Can you work these out from the model? Positions are in its coordinate system, mm. A direction names the side the tool comes from. Give positions to 0.01 mm unless a question says otherwise; leave off trailing zeros. Loops run counter-clockwise (first coordinate to the right, second up) from the corner with the lowest first, then second, coordinate; pieces in that order, holes last. Notation, with made-up numbers: (44, 63) - (51, 63) arc R16 cw to (51, 76) - close; hole circle Ø7 at (31, 9). An arc over 180 degrees is marked (long way). Answer in a Markdown table with one row per item.
from build123d import *

# Parameters (mm, degrees)
BOSS_EXTRUDE1_DEPTH  = 21
SKETCH2_R            = 1.825
CUT_EXTRUDE1_DEPTH   = 4
SKETCH3_W            = 7.5
SKETCH3_H            = 11.75
CUT_EXTRUDE2_DEPTH   = 13
FILLET1_R            = 4
SKETCH5_R            = 1.825
CUT_EXTRUDE3_DEPTH   = 41.522370365
FILLET1_OF_MIRROR1_R = 4


with BuildPart() as part:
    # Sketch1 → Boss-Extrude1 (new body)
    with BuildSketch(Plane(origin=(0, 0, 0), x_dir=(1, 0, 0), z_dir=(0, 1, 0))):
        Polygon((-24.5, 0), (-24.5, 12.75), (0, 12.75), (0, 15.75), (-35, 15.75), (-35, 0), align=None)
    boss_extrude1 = extrude(amount=BOSS_EXTRUDE1_DEPTH)

    # Sketch2 → Cut-Extrude1 (cut)
    with BuildSketch(Plane.XY):
        with Locations((-31.25, 7)):
            Circle(SKETCH2_R)
    cut_extrude1 = extrude(amount=-CUT_EXTRUDE1_DEPTH, mode=Mode.SUBTRACT)

    # Sketch3 → Cut-Extrude2 (cut)
    with BuildSketch(Plane.XZ):
        with Locations((-31.25, -9.875)):
            Rectangle(SKETCH3_W, SKETCH3_H)
    cut_extrude2 = extrude(amount=-CUT_EXTRUDE2_DEPTH, mode=Mode.SUBTRACT)

    # Fillet1
    fillet1_edges = [part.edges().sort_by_distance(p)[0] for p in [
        (-35, 17, -15.75),
    ]]
    fillet(fillet1_edges, radius=FILLET1_R)

    # Sketch5 → Cut-Extrude3 (cut, through all)
    with BuildSketch(Plane.XZ.offset(-13)):
        with Locations(Location((-31, -11.75, 0), (0, 0, 270))):
            Circle(SKETCH5_R)
    cut_extrude3 = extrude(amount=-CUT_EXTRUDE3_DEPTH, mode=Mode.SUBTRACT)

    # Mirror1: Boss-Extrude1, Cut-Extrude1, Cut-Extrude2, Cut-Extrude3 across plane
    add(boss_extrude1.mirror(Plane(origin=(0, 21, 0), x_dir=(0, 0, 1), z_dir=(-1, 0, 0))))
    add(cut_extrude1.mirror(Plane(origin=(0, 21, 0), x_dir=(0, 0, 1), z_dir=(-1, 0, 0))), mode=Mode.SUBTRACT)
    add(cut_extrude2.mirror(Plane(origin=(0, 21, 0), x_dir=(0, 0, 1), z_dir=(-1, 0, 0))), mode=Mode.SUBTRACT)
    add(cut_extrude3.mirror(Plane(origin=(0, 21, 0), x_dir=(0, 0, 1), z_dir=(-1, 0, 0))), mode=Mode.SUBTRACT)

    # Fillet1 of Mirror1
    fillet1_of_mirror1_edges = [part.edges().sort_by_distance(p)[0] for p in [
        (35, 17, -15.75),
    ]]
    fillet(fillet1_of_mirror1_edges, radius=FILLET1_OF_MIRROR1_R)


solid = part.part
Q1. If we mould it in two halves opening along X, with no side actions, what happens to faces 1 (the face through (30, 10, 0)), 2 (the face through (29.77, 16.94, -10.4)), 3 (the face through (35, 13, -3))? For each: released by +X, released by -X, zero draft, split by the parting line, or undercut.
Checked values:
| item | result |
|---|---|
| face 1 | zero draft |
| face 2 | undercut |
| face 3 | released by +X |
Q2. Imagine slicing it at A-A, the plane z = -2.5. Write out the boundary of the cut face in (x, y) (3 decimals), and give its area (3 significant figures).
Checked values:
| item | result |
|---|---|
| outline | (-35, 0) - (-24.5, 0) - (-24.5, 21) - (-35, 21) - close; (24.5, 0) - (35, 0) - (35, 21) - (24.5, 21) - close; hole circle Ø3.65 at (-31.25, 7); hole circle Ø3.65 at (31.25, 7) |
| area | 420 mm² |
Q3. For pin 1 (2 mm diameter, centred on x = 32, z = -9.5, fed in from -Y); pin 2 (4.5 mm diameter, centred on x = 31.25, y = 7, fed in from -Z); pin 3 (8 mm diameter, centred on x = 7, y = 5.5, fed in from +Z); pin 4 (1 mm diameter, centred on x = 14.5, z = -12, fed in from +Y), each with a flat end and sliding along its axis, tell me the tip position at first contact or that it passes through.
Checked values:
| item | result |
|---|---|
| pin 1 | stops at y = 13 |
| pin 2 | stops at z = -4 |
| pin 3 | stops at z = -12.75 |
| pin 4 | passes through |
Q4. Imagine slicing it at C-C, the plane y = 10.25. Write out the boundary of the cut face in (x, z), and give its area (4 significant figures).
Checked values:
| item | result |
|---|---|
| outline | (-35, -4) - (-27.5, -4) - (-27.5, -15.75) - (27.5, -15.75) - (27.5, -4) - (35, -4) - (35, 0) - (24.5, 0) - (24.5, -12.75) - (-24.5, -12.75) - (-24.5, 0) - (-35, 0) - close |
| area | 301.5 mm² |
Q5. If I drill on line 1 (X direction, y = 16.5, z = -11.75) (3 decimals); line 2 (Y direction, x = -31.25, z = -1.8) (3 decimals); line 3 (X direction, y = 2.5, z = -6.5), over which ranges is the centre line in solid material (lowest first)? Write a range as [from, to].
Checked values:
| item | result |
|---|---|
| line 1 | x = [-35, -32.825], [-29.175, -24.5], [24.5, 29.175], [32.825, 35] |
| line 2 | y = [0, 5.175], [8.825, 21] |
| line 3 | x = [-27.5, -24.5], [24.5, 27.5] |
Q6. Imagine slicing it at D-D, the plane y = 18.5. Write out the boundary of the cut face in (x, z) (3 decimals), and give its area (3 significant figures).
Checked values:
| item | result |
|---|---|
| outline | (-35, -11.75) arc R4 ccw to (-31, -15.75) - (31, -15.75) arc R4 ccw to (35, -11.75) - (35, 0) - (24.5, 0) - (24.5, -12.75) - (-24.5, -12.75) - (-24.5, 0) - (-35, 0) - close; hole circle Ø3.65 at (-31, -11.75); hole circle Ø3.65 at (31, -11.75) |
| area | 450 mm² |
Q7. On a 3-axis mill with a long thin cutter (end or side, diameter ignored), from which of +Z, -Z, +X, -X, +Y, -Y can I reach the whole of each face in a straight line? I mean faces 4 (the face through (-35, 13, -3)), 5 (the face through (31, 5, -4)), 6 (the face through (-30.27, 8.54, -1.97)), 7 (the face through (-31.3, 13, -9.79)), 8 (the face through (-24.5, 10, -6)). Say none if no direction works.
Checked values:
| item | result |
|---|---|
| face 4 | +Z, -Z, -X, +Y, -Y |
| face 5 | -Z, +X, -Y |
| face 6 | +Z, -Z |
| face 7 | -Z, -X, -Y |
| face 8 | +Z, +Y, -Y |
Q8. Imagine slicing it at B-B, the plane z = -6. Write out the boundary of the cut face in (x, y).
Checked values:
| item | result |
|---|---|
| outline | (-35, 13) - (-27.5, 13) - (-27.5, 0) - (-24.5, 0) - (-24.5, 21) - (-35, 21) - close; (24.5, 0) - (27.5, 0) - (27.5, 13) - (35, 13) - (35, 21) - (24.5, 21) - close |
